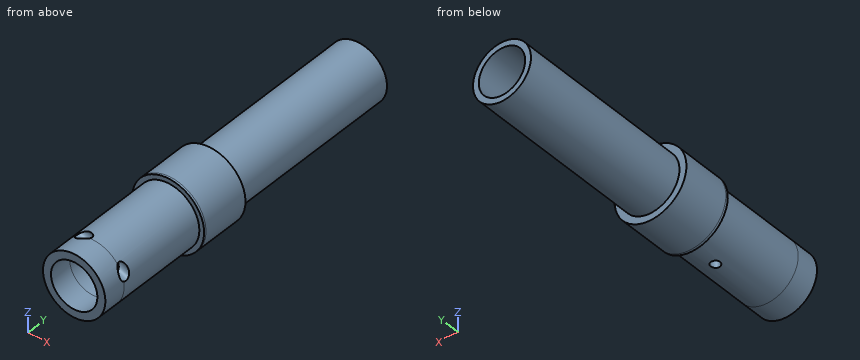
from build123d import *
from build123d.topology import SkipClean

# Parameters (mm, degrees)
SKETCH1_R                = 13.45
SKETCH1_R_2              = 10
BOSS_EXTRUDE1_DEPTH      = 100
BOSS_EXTRUDE2_DEPTH      = 85
BOSS_EXTRUDE2_DEPTH_BACK = 4
SKETCH6_R                = 12.5
SKETCH6_R_2              = 10
BOSS_EXTRUDE3_START      = -84
SKETCH7_R                = 15.5
SKETCH7_R_2              = 10
BOSS_EXTRUDE3_DEPTH      = 1
CUT_EXTRUDE1_DEPTH       = 187.294122291
CUT_EXTRUDE1_DEPTH_BACK  = 187.294122291
SKETCH11_W               = 35.010034018
SKETCH11_H               = 2.4
CUT_EXTRUDE3_DEPTH       = 187.294122291
CUT_EXTRUDE3_DEPTH_BACK  = 187.294122291
SKETCH13_W               = 32.559051685
SKETCH13_H               = 42.8
SKETCH14_R               = 15.5
BOSS_EXTRUDE4_DEPTH      = 21
SKETCH15_R               = 10
CUT_EXTRUDE4_DEPTH       = 22
BOSS_EXTRUDE5_START      = 10
SKETCH17_R               = 13.45
SKETCH17_R_2             = 10
BOSS_EXTRUDE5_DEPTH      = 10
SKETCH18_R               = 2.5
CUT_EXTRUDE5_DEPTH       = 54
SKETCH20_R               = 2
CUT_EXTRUDE6_DEPTH       = 22


with BuildPart() as part:
    # Sketch1 → Boss-Extrude1 (new body)
    with BuildSketch(Plane(origin=(0, 0, 0), x_dir=(1, 0, 0), z_dir=(0, 1, 0))):
        with Locations(Location((0, 0, 0), (0, 0, 270))):
            Circle(SKETCH1_R)
        with Locations(Location((0, 0, 0), (0, 0, 270))):
            Circle(SKETCH1_R_2, mode=Mode.SUBTRACT)
    extrude(amount=BOSS_EXTRUDE1_DEPTH)

    # Sketch6 → Boss-Extrude2 (add, two sides: drawn at the far end of the back side and taken through both)
    with BuildSketch(Plane(origin=(0, 100, 0), x_dir=(1, 0, 0), z_dir=(0, 1, 0)).offset(-BOSS_EXTRUDE2_DEPTH_BACK)):
        with Locations(Location((0, 0, 0), (0, 0, 270))):
            Circle(SKETCH6_R)
        with Locations(Location((0, 0, 0), (0, 0, 270))):
            Circle(SKETCH6_R_2, mode=Mode.SUBTRACT)
    extrude(amount=BOSS_EXTRUDE2_DEPTH + BOSS_EXTRUDE2_DEPTH_BACK)

    # Sketch7 → Boss-Extrude3 (add)
    with BuildSketch(Plane.XZ.offset(BOSS_EXTRUDE3_START)):
        with Locations(Location((0, 0, 0), (0, 0, 270))):
            Circle(SKETCH7_R)
        with Locations(Location((0, 0, 0), (0, 0, 90))):
            Circle(SKETCH7_R_2, mode=Mode.SUBTRACT)
    extrude(amount=-BOSS_EXTRUDE3_DEPTH)

    # Sketch11 → Cut-Extrude1 (cut, two sides: drawn at the far end of the back side and taken through both)
    with BuildSketch(Plane(origin=(0, 0, 0), x_dir=(0, 0, -1), z_dir=(1, 0, 0)).offset(-CUT_EXTRUDE1_DEPTH_BACK)):
        Rectangle(SKETCH11_W, SKETCH11_H)
    extrude(amount=CUT_EXTRUDE1_DEPTH + CUT_EXTRUDE1_DEPTH_BACK, mode=Mode.SUBTRACT)

    # Sketch13 → Cut-Extrude3 (cut, two sides: drawn at the far end of the back side and taken through both)
    with BuildSketch(Plane.XY.offset(-CUT_EXTRUDE3_DEPTH_BACK)):
        with Locations((2.829525842, 22.6)):
            Rectangle(SKETCH13_W, SKETCH13_H)
    extrude(amount=CUT_EXTRUDE3_DEPTH + CUT_EXTRUDE3_DEPTH_BACK, mode=Mode.SUBTRACT)

    # Sketch14 → Boss-Extrude4 (add)
    with BuildSketch(Plane(origin=(0, 85, 0), x_dir=(1, 0, 0), z_dir=(0, 1, 0))):
        with Locations(Location((0, 0, 0), (0, 0, 270))):
            Circle(SKETCH14_R)
    extrude(amount=BOSS_EXTRUDE4_DEPTH)

    # Sketch15 → Cut-Extrude4 (cut)
    with BuildSketch(Plane.XZ.offset(-85)):
        with Locations(Location((0, 0, 0), (0, 0, 90))):
            Circle(SKETCH15_R)
    extrude(amount=-CUT_EXTRUDE4_DEPTH, mode=Mode.SUBTRACT)

    # Sketch17 → Boss-Extrude5 (add)
    with BuildSketch(Plane.XZ.offset(-44).offset(BOSS_EXTRUDE5_START)):
        with Locations(Location((0, 0, 0), (0, 0, 270))):
            Circle(SKETCH17_R)
        with Locations(Location((0, 0, 0), (0, 0, 270))):
            Circle(SKETCH17_R_2, mode=Mode.SUBTRACT)
    extrude(amount=-BOSS_EXTRUDE5_DEPTH)

    # Sketch18 → Cut-Extrude5 (cut)
    with SkipClean():  # the faces are left unmerged after this step: merging them gives an invalid solid
        with BuildSketch(Plane(origin=(35.019010809, 0, -14.753605728), x_dir=(-0.38825278231327914, 1.212401304802914e-15, -0.9215529160205601), z_dir=(0.9215529160205602, -2.877743595734803e-15, -0.3882527823132792))):
            with Locations((-9.45, 45)):
                Circle(SKETCH18_R)
        extrude(amount=-CUT_EXTRUDE5_DEPTH, mode=Mode.SUBTRACT)

    # Sketch20 → Cut-Extrude6 (cut)
    with BuildSketch(Plane.XY):
        with Locations(Location((0, 71.5, 0), (0, 0, 90))):
            Circle(SKETCH20_R)
    extrude(amount=-CUT_EXTRUDE6_DEPTH, mode=Mode.SUBTRACT)


solid = part.part
The model under review builds one solid part; all positions refer to its coordinate system, in mm. Give positions to 0.01 mm unless a question says otherwise; leave off trailing zeros. Order: outer loops, then holes, each group sorted by start corner. A loop starts at its lowest first (then second) coordinate and runs counter-clockwise, first axis right, second up. Notation, with made-up numbers: M -21.75,5.25 L 6.25,5.25 A33 cw 6.25,39.25 Z; hole C 88.25,5 d9. An arc over 180 degrees is marked long. Answer in a Markdown table with one row per item. Add a question column.
1. To check wall thickness, follow line 1 along X through (y, z) = (69, 0); line 2 along X through (y, z) = (99, 0); line 3 along Z through (x, y) = (0, 166). State the ranges of each line that lie inside material, in increasing order.
2. Add section A-A on z = 0. State the section outline as (x, y) points, plus the area to 3 significant figures.
3. Add section C-C on x = 0. Count the separate pieces of the cut face and the enclosed holes in it, plus the area to 3 significant figures.
4. For pin 1 Ø8 at (y, z) = (62.5, 12) entering from -X; pin 2 Ø2 at (y, z) = (136.5, -7.5) entering from -X; pin 3 Ø5 at (x, y) = (0, 71.5) entering from -Z, all flat-tipped, find the tip position at first contact; note any pin that passes through.
5. Add section B-B on y = 88.5. State the section outline as (x, z) points, plus the area to 3 significant figures.
6. Add section D-D on y = 119. State the section outline as (x, z) points.
The answers:
| question | item | result |
|---|---|---|
| 1 | line 1 | -13.45 to -10, 10 to 13.45 |
| 1 | line 2 | -15.5 to -10, 10 to 15.5 |
| 1 | line 3 | -12.5 to -10, 10 to 12.5 |
| 2 | outline | M -15.5,84 L -13.45,84 L -13.45,34 L -10,34 L -10,185 L -12.5,185 L -12.5,106 L -15.5,106 Z; M 10,34 L 13.45,34 L 13.45,84 L 15.5,84 L 15.5,106 L 12.5,106 L 12.5,185 L 10,185 Z |
| 2 | area | 982 mm2 |
| 3 | separate pieces | 3 |
| 3 | enclosed holes | 0 |
| 3 | area | 956 mm2 |
| 4 | pin 1 | x = -10.81 |
| 4 | pin 2 | x = -10.68 |
| 4 | pin 3 | z = -13.45 |
| 5 | outline | C 0,0 d31; hole C 0,0 d20 |
| 5 | area | 441 mm2 |
| 6 | outline | C 0,0 d25; hole C 0,0 d20 |
